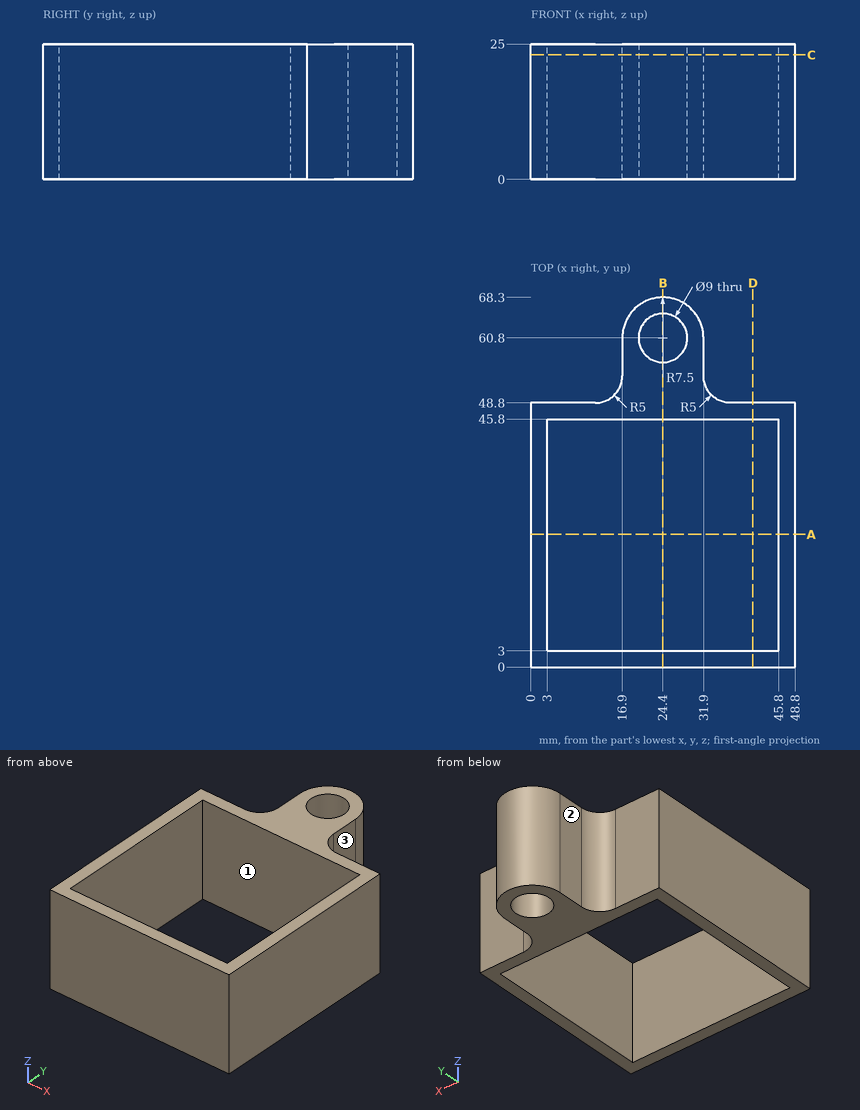
Print and shaded views of the part. All mm, measured from the part's lowest x, y and z. A direction names the side the tool comes from. Coordinates: 2 decimals unless noted, no trailing zeros. Order: outer loops, then holes, each group sorted by start corner. A loop starts at its lowest first (then second) coordinate and runs counter-clockwise, first axis right, second up. Notation, with made-up numbers: M -14.75,-33 L 33.25,-33 A25 ccw 33.25,2 Z; hole C 8.25,33.25 d1. An arc over 180 degrees is marked long. One line per question, with ' | ' between items. Start each with the question number.
Q1. 3-axis set-ups, long thin cutter, end or side, ignore diameter. For the marked faces 1, 2 and 3: which of +Z, -Z, +X, -X, +Y, -Y reach the whole face in a straight line?
Q2. Flat gauge pins, fed straight in: pin 1 Ø3 at (x, z) = (14.5, 13.5) entering from +Y; pin 2 Ø9.5 at (x, z) = (45, 7) entering from +Y; pin 3 Ø5.5 at (y, z) = (56.5, 10.5) entering from +X. Where does each tip first touch, or does it go through?
Q3. Saw through at B-B (x = 24.4). List the corners of the cut face in (y, z).
Q4. Saw through at A-A (y = 24.5). List the corners of the cut face in (x, z), then the cut area to 3 significant figures.
Q5. Saw through at C-C (z = 23). List the corners of the cut face in (x, y).
Q6. Probe L1, parallel to Y at x = 24.4, z = 19.75; L2, parallel to X at y = 17, z = 8. List the from-to ranges inside material, lowest first. Write a range as from..to.
Check values:
1) face 1: +Z, -Z | face 2: +Z, -Z, -X, +Y | face 3: +Z, -Z, +X, +Y
2) pin 1: stops at y = 50.94 | pin 2: stops at y = 48.8 | pin 3: stops at x = 31.9
3) outline: M 0,0 L 3,0 L 3,25 L 0,25 Z; M 45.8,0 L 56.3,0 L 56.3,25 L 45.8,25 Z; M 65.3,0 L 68.3,0 L 68.3,25 L 65.3,25 Z
4) outline: M 0,0 L 3,0 L 3,25 L 0,25 Z; M 45.8,0 L 48.8,0 L 48.8,25 L 45.8,25 Z | area: 150 mm2
5) outline: M 0,0 L 48.8,0 L 48.8,48.8 L 36.9,48.8 A5 cw 31.9,53.8 L 31.9,60.8 A7.5 ccw 16.9,60.8 L 16.9,53.8 A5 cw 11.9,48.8 L 0,48.8 Z; hole M 3,3 L 45.8,3 L 45.8,45.8 L 3,45.8 Z; hole C 24.4,60.8 d9
6) L1: y = 0..3, 45.8..56.3, 65.3..68.3 | L2: x = 0..3, 45.8..48.8
